from build123d import *

# Parameters (mm, degrees)
SKETCH1_R           = 75
BOSS_EXTRUDE1_DEPTH = 10


with BuildPart() as part:
    # Sketch1 → Boss-Extrude1 (new, symmetric)
    with BuildSketch(Plane.XY):
        Circle(SKETCH1_R)
        with BuildLine():
            Line((-5, 46.314144708), (-5, 45))
            Line((-5, 45), (5, 45))
            Line((5, 45), (5, 46.314144708))
            ThreePointArc((5, 46.314144708), (6.067632914, 48.608912113), (8.510638298, 49.27036671))
            ThreePointArc((8.510638298, 49.27036671), (35.355339059, 35.355339059), (49.27036671, 8.510638298))
            ThreePointArc((49.27036671, 8.510638298), (48.608912113, 6.067632914), (46.314144708, 5))
            Line((46.314144708, 5), (45, 5))
            Line((45, 5), (45, -5))
            Line((45, -5), (46.314144708, -5))
            ThreePointArc((46.314144708, -5), (48.608912113, -6.067632914), (49.27036671, -8.510638298))
            ThreePointArc((49.27036671, -8.510638298), (35.355339059, -35.355339059), (8.510638298, -49.27036671))
            ThreePointArc((8.510638298, -49.27036671), (6.067632914, -48.608912113), (5, -46.314144708))
            Line((5, -46.314144708), (5, -45))
            Line((5, -45), (-5, -45))
            Line((-5, -45), (-5, -46.314144708))
            ThreePointArc((-5, -46.314144708), (-6.067632914, -48.608912113), (-8.510638298, -49.27036671))
            ThreePointArc((-8.510638298, -49.27036671), (-35.355339059, -35.355339059), (-49.27036671, -8.510638298))
            ThreePointArc((-49.27036671, -8.510638298), (-48.608912113, -6.067632914), (-46.314144708, -5))
            Line((-46.314144708, -5), (-45, -5))
            Line((-45, -5), (-45, 5))
            Line((-45, 5), (-46.314144708, 5))
            ThreePointArc((-46.314144708, 5), (-48.608912113, 6.067632914), (-49.27036671, 8.510638298))
            ThreePointArc((-49.27036671, 8.510638298), (-35.355339059, 35.355339059), (-8.510638298, 49.27036671))
            ThreePointArc((-8.510638298, 49.27036671), (-6.067632914, 48.608912113), (-5, 46.314144708))
        make_face(mode=Mode.SUBTRACT)
    extrude(amount=BOSS_EXTRUDE1_DEPTH, both=True)


solid = part.part
Source: CAD feature listing. Evaluate the final solid. Frame: model axes, mm. A direction names the side the tool comes from. Coordinates: 2 decimals unless noted, no trailing zeros. Loops run counter-clockwise (first coordinate to the right, second up) from the corner with the lowest first, then second, coordinate; pieces in that order, holes last. Notation, with made-up numbers: (70.25, 49) - (129.25, 49) arc R19 cw to (129.25, 67) - close; hole circle Ø6 at (67.5, 25). An arc over 180 degrees is marked (long way). One line per question, with ' | ' between items.
1) Section D-D, the plane x = 60.5. Return loops of the section in (y, z), then the cut area to 3 significant figures.
Report:
outline: (-44.33, -10) - (44.33, -10) - (44.33, 10) - (-44.33, 10) - close | area: 1,770 mm²
2) Section A-A, the plane y = 0. Return loops of the section in (x, z).
Report:
outline: (-75, -10) - (-45, -10) - (-45, 10) - (-75, 10) - close; (45, -10) - (75, -10) - (75, 10) - (45, 10) - close
3) Pull-direction query (X, two-part tool) for faces 1 (the face through (35.66, -35.05, 0.14)), 2 (the face through (-9.764, 74.362, 0.14)), 3 (the face through (-6.04, -48.585, 0.14)), 4 (the face through (49, 1, -10)); classes: released by +X, released by -X, zero draft, split by the parting line, or undercut.
Report:
face 1: undercut | face 2: split by the parting line | face 3: undercut | face 4: zero draft
4) Set-up query: faces 5 (the face through (-45, 0, 0)), 6 (the face through (49, 1, 10)). Return all of +Z, -Z, +X, -X, +Y, -Y with unobstructed straight access to the full face (end or side cutting, diameter ignored); none if empty.
Report:
face 5: +Z, -Z | face 6: +Z, +X, -X, +Y, -Y
5) Section C-C, the plane z = -7.25. Return loops of the section in (x, y), then the cut area to 3 significant figures.
Report:
outline: circle Ø150 at (0, 0); hole (-49.27, -8.51) arc R50 ccw to (-8.51, -49.27) arc R3 ccw to (-5, -46.31) - (-5, -45) - (5, -45) - (5, -46.31) arc R3 ccw to (8.51, -49.27) arc R50 ccw to (49.27, -8.51) arc R3 ccw to (46.31, -5) - (45, -5) - (45, 5) - (46.31, 5) arc R3 ccw to (49.27, 8.51) arc R50 ccw to (8.51, 49.27) arc R3 ccw to (5, 46.31) - (5, 45) - (-5, 45) - (-5, 46.31) arc R3 ccw to (-8.51, 49.27) arc R50 ccw to (-49.27, 8.51) arc R3 ccw to (-46.31, 5) - (-45, 5) - (-45, -5) - (-46.31, -5) arc R3 ccw to start | area: 10,000 mm²
6) Line query: line 1 along Y through (x, z) = (46, -1.75); line 2 along Y through (x, z) = (0, -7.5); line 3 along Y through (x, z) = (3.5, 4.5). Output: solid intervals per line, ascending.
Report:
line 1: y = -59.24 to -19.6, -5 to 5, 19.6 to 59.24 | line 2: y = -75 to -45, 45 to 75 | line 3: y = -74.92 to -45, 45 to 74.92
7) Section B-B, the plane x = 11. Return loops of the section in (y, z) (3 decimals), then the cut area to 3 significant figures.
Report:
outline: (-74.189, -10) - (-48.775, -10) - (-48.775, 10) - (-74.189, 10) - close; (48.775, -10) - (74.189, -10) - (74.189, 10) - (48.775, 10) - close | area: 1,020 mm²
8) First-contact query: P1, Ø8, axis at x = 2, z = -8, coming from the -Y side; P2, Ø3, axis at y = -4.5, z = 5, coming from the +X side; P3, Ø1.5, axis at x = 20, z = 2.5, coming from the +Y side. Flat tips, straight axial feed; report the tip coordinate or a pass-through.
Report:
P1: stops at y = -75 | P2: stops at x = 74.94 | P3: stops at y = 72.49
